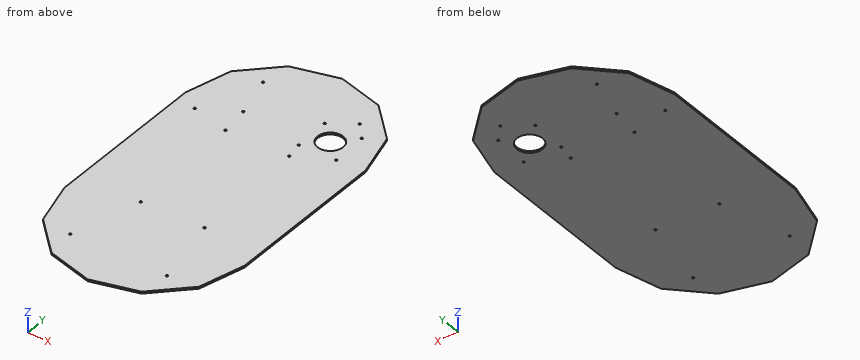
from build123d import *

# Parameters (mm, degrees)
F1_DEPTH = 3.175
F2_R     = 20.6375
F2_R_2   = 1.7272
F3_DEPTH = 3.175


with BuildPart() as f1:
    # F0 (on Top) → F1 (new body)
    with BuildSketch(Plane.XY):
        Polygon((292.1, -265.154105), (292.1, 0), (272.53301, 73.025), (219.075, 126.48301), (146.05, 146.05), (73.025, 126.48301), (19.56699, 73.025), (0, 0), (0, -265.154105), (19.56699, -338.179105), (73.025, -391.637115), (146.05, -411.204105), (219.075, -391.637115), (272.53301, -338.179105), align=None)
    extrude(amount=F1_DEPTH)

    # F2 (on face) → F3 (cut, through all)
    with BuildSketch(Plane.XY.offset(3.175)):
        with Locations((217.185523, 23.698288)):
            Circle(F2_R)
        with Locations((92.312386, -37.126894)):
            Circle(F2_R_2)
        with Locations((193.443454, -33.823195)):
            Circle(F2_R_2)
        with Locations((188.791324, -6.613696)):
            Circle(F2_R_2)
        with Locations((247.497507, -4.695911)):
            Circle(F2_R_2)
        with Locations((245.579723, 54.010272)):
            Circle(F2_R_2)
        with Locations((186.873539, 52.092488)):
            Circle(F2_R_2)
        with Locations((199.787614, -228.027211)):
            Circle(F2_R_2)
        with Locations((98.656546, -231.330911)):
            Circle(F2_R_2)
        with Locations((224.475897, 78.425897)):
            Circle(F2_R_2)
        with Locations((67.624103, 78.425897)):
            Circle(F2_R_2)
        with Locations((67.624103, -343.580002)):
            Circle(F2_R_2)
        with Locations((224.475897, -343.580002)):
            Circle(F2_R_2)
        with Locations((31.05851, -21.485911)):
            Circle(F2_R_2)
        with Locations((86.051124, 10.264089)):
            Circle(F2_R_2)
    extrude(amount=-F3_DEPTH, mode=Mode.SUBTRACT)


solid = f1.part
Input: part model. Units: mm. Frame: model coordinates. Round coordinates to 2 decimals unless told otherwise and drop trailing zeros. Order: outer loops, then holes, each group sorted by start corner. A loop starts at its lowest first (then second) coordinate and runs counter-clockwise, first axis right, second up.
1. Cut plane B-B, the plane z = 1.25. State how many separate pieces and enclosed holes the cut face has, then the cut area to 3 significant figures.
The answers:
separate pieces: 1
enclosed holes: 15
area: 140,000 mm2
2. Material intervals for line 1 (Y direction, x = 188, z = 2.3); line 2 (Y direction, x = 235, z = 2); line 3 (X direction, y = -7, z = 2.55), sorted ascending.
The answers:
line 1: y = -399.96 to -8.15, -5.08 to 50.78, 53.4 to 134.81
line 2: y = -375.71 to 13.28, 34.12 to 110.56
line 3: x = 0 to 187.11, 190.47 to 292.1
3. Cut plane C-C, the plane y = 31. Output: boundary loops of the cut face in (x, z) (3 decimals).
The answers:
outline: (8.306, 0) - (197.883, 0) - (197.883, 3.175) - (8.306, 3.175) - close; (236.488, 0) - (283.794, 0) - (283.794, 3.175) - (236.488, 3.175) - close
4. Cut plane A-A, the plane x = 209. Output: boundary loops of the cut face in (y, z) (3 decimals), then the cut area to 3 significant figures.
The answers:
outline: (-394.337, 0) - (4.754, 0) - (4.754, 3.175) - (-394.337, 3.175) - close; (42.643, 0) - (129.183, 0) - (129.183, 3.175) - (42.643, 3.175) - close
area: 1,540 mm2
5. Pin query (flat end, axial travel): P1, Ø2, axis at x = 31.06, y = -21.49, coming from the -Z side; P2, Ø1, axis at y = -288.5, z = 2, coming from the -X side. Return the tip coordinate at first contact, or that it passes through.
The answers:
P1: passes through
P2: stops at x = 6.12
6. Cut plane D-D, the plane y = 111.5. Output: boundary loops of the cut face in (x, z) (3 decimals).
The answers:
outline: (58.042, 0) - (234.058, 0) - (234.058, 3.175) - (58.042, 3.175) - close
